Geometry: final body of the model. Coordinates: model frame, mm. Round coordinates to 2 decimals unless told otherwise and drop trailing zeros. Loops run counter-clockwise (first coordinate to the right, second up) from the corner with the lowest first, then second, coordinate; pieces in that order, holes last. Notation, with made-up numbers: M 69,-26 L 83,-26 A8 cw 83,-20 Z; hole C 15.25,-26.5 d6. An arc over 180 degrees is marked long. Return JSON: item names as keys, results as strings.
from build123d import *

# Parameters (mm, degrees)
F0_R        = 51.2
F1_DEPTH    = 1.5
F2_T1_DEPTH = 3
F3_R        = 5.08


# Not quite as in the source:
# - a fillet or chamfer that OpenCascade refuses, or shapes differently, is made with other operations: its cross-section is extruded or revolved along the edge and cut away or added


with BuildPart() as f1:
    # F0 (on Front) → F1 (new body, symmetric)
    with BuildSketch(Plane.XZ):
        Circle(F0_R)
        with BuildLine():
            ThreePointArc((1.5, 44.1745401787), (25.9801081513, 35.7585511514), (41.5489587997, 15.0772684084))
            ThreePointArc((41.5489587997, 15.0772684084), (42.0366980202, 13.6585511514), (42.4760097829, 12.2240988595))
            ThreePointArc((42.4760097829, 12.2240988595), (43.7668803572, 6.1725346333), (44.2, 0))
            ThreePointArc((44.2, 0), (39.7173586616, -19.3951391062), (27.1786687354, -34.8562758448))
            ThreePointArc((27.1786687354, -34.8562758448), (25.9801081513, -35.7585511514), (24.7516177523, -36.6196316017))
            ThreePointArc((24.7516177523, -36.6196316017), (0, -44.2), (-24.7516177523, -36.6196316017))
            ThreePointArc((-24.7516177523, -36.6196316017), (-25.9801081513, -35.7585511514), (-27.1786687354, -34.8562758448))
            ThreePointArc((-27.1786687354, -34.8562758448), (-42.0366980202, -13.6585511514), (-42.4760097829, 12.2240988595))
            ThreePointArc((-42.4760097829, 12.2240988595), (-42.0366980202, 13.6585511514), (-41.5489587997, 15.0772684084))
            ThreePointArc((-41.5489587997, 15.0772684084), (-25.9801081513, 35.7585511514), (-1.5, 44.1745401787))
            ThreePointArc((-1.5, 44.1745401787), (0, 44.2), (1.5, 44.1745401787))
        make_face(mode=Mode.SUBTRACT)
        with BuildLine():
            Line((-24.7516177523, -36.6196316017), (-1.118469097, -4.8732973313))
            ThreePointArc((-1.118469097, -4.8732973313), (-2.9389262615, -4.0450849719), (-4.2891552241, -2.569659017))
            Line((-4.2891552241, -2.569659017), (-27.1786687354, -34.8562758448))
            ThreePointArc((-27.1786687354, -34.8562758448), (-25.9801081513, -35.7585511514), (-24.7516177523, -36.6196316017))
        make_face()
        with BuildLine():
            ThreePointArc((-4.9804071414, -0.4422043711), (-4.7552825815, 1.5450849719), (-3.7693128085, 3.2851607193))
            Line((-3.7693128085, 3.2851607193), (-41.5489587997, 15.0772684084))
            ThreePointArc((-41.5489587997, 15.0772684084), (-42.0366980202, 13.6585511514), (-42.4760097829, 12.2240988595))
            Line((-42.4760097829, 12.2240988595), (-4.9804071414, -0.4422043711))
        make_face()
        with BuildLine():
            ThreePointArc((-1.9595917942, 4.6), (0, 5), (1.9595917942, 4.6))
            Line((1.9595917942, 4.6), (1.5, 44.1745401787))
            ThreePointArc((1.5, 44.1745401787), (0, 44.2), (-1.5, 44.1745401787))
            Line((-1.5, 44.1745401787), (-1.9595917942, 4.6))
        make_face()
        with BuildLine():
            ThreePointArc((3.7693128085, 3.2851607193), (4.6822304537, 1.7540575757), (5, 0))
            ThreePointArc((5, 0), (4.9950993837, -0.2213191055), (4.9804071414, -0.4422043711))
            Line((4.9804071414, -0.4422043711), (42.4760097829, 12.2240988595))
            ThreePointArc((42.4760097829, 12.2240988595), (42.0366980202, 13.6585511514), (41.5489587997, 15.0772684084))
            Line((41.5489587997, 15.0772684084), (3.7693128085, 3.2851607193))
        make_face()
        with BuildLine():
            Line((27.1786687354, -34.8562758448), (4.2891552241, -2.569659017))
            ThreePointArc((4.2891552241, -2.569659017), (2.9389262615, -4.0450849719), (1.118469097, -4.8732973313))
            Line((1.118469097, -4.8732973313), (24.7516177523, -36.6196316017))
            ThreePointArc((24.7516177523, -36.6196316017), (25.9801081513, -35.7585511514), (27.1786687354, -34.8562758448))
        make_face()
        with BuildLine():
            ThreePointArc((4.9804071414, -0.4422043711), (4.9950993837, -0.2213191055), (5, 0))
            ThreePointArc((5, 0), (4.6822304537, 1.7540575757), (3.7693128085, 3.2851607193))
            ThreePointArc((3.7693128085, 3.2851607193), (2.9389262615, 4.0450849719), (1.9595917942, 4.6))
            ThreePointArc((1.9595917942, 4.6), (0, 5), (-1.9595917942, 4.6))
            ThreePointArc((-1.9595917942, 4.6), (-2.9389262615, 4.0450849719), (-3.7693128085, 3.2851607193))
            ThreePointArc((-3.7693128085, 3.2851607193), (-4.7552825815, 1.5450849719), (-4.9804071414, -0.4422043711))
            ThreePointArc((-4.9804071414, -0.4422043711), (-4.7552825815, -1.5450849719), (-4.2891552241, -2.569659017))
            ThreePointArc((-4.2891552241, -2.569659017), (-2.9389262615, -4.0450849719), (-1.118469097, -4.8732973313))
            ThreePointArc((-1.118469097, -4.8732973313), (0, -5), (1.118469097, -4.8732973313))
            ThreePointArc((1.118469097, -4.8732973313), (2.9389262615, -4.0450849719), (4.2891552241, -2.569659017))
            ThreePointArc((4.2891552241, -2.569659017), (4.7552825815, -1.5450849719), (4.9804071414, -0.4422043711))
        make_face()
        with BuildLine():
            ThreePointArc((0, 1.5), (1.0606601718, 1.0606601718), (1.5, 0))
            ThreePointArc((1.5, 0), (-1.0606601718, -1.0606601718), (0, 1.5))
        make_face(mode=Mode.SUBTRACT)
    extrude(amount=F1_DEPTH, both=True)

    # F2: fillet of radius 3 on 10 edges, made by hand

    # F2_s2 → F2_t1 (join)
    with BuildSketch(Plane.XZ.offset(-1.5)):
        with BuildLine():
            ThreePointArc((3.0875868977, 3.9327861815), (2.2498717307, 4.9648804635), (1.9403413197, 6.2576202799))
            Line((1.9403413197, 6.2576202799), (1.9595917942, 4.6))
            ThreePointArc((1.9595917942, 4.6), (2.5455444913, 4.303510572), (3.0875868977, 3.9327861815))
        make_face()
        with BuildLine():
            ThreePointArc((2.7861851021, 4.151767404), (4.0266333175, 3.6739876086), (5.351752101, 3.7790852667))
            Line((5.351752101, 3.7790852667), (3.7693128085, 3.2851607193))
            ThreePointArc((3.7693128085, 3.2851607193), (3.3062652647, 3.7508145781), (2.7861851021, 4.151767404))
        make_face()
        with BuildLine():
            ThreePointArc((-2.7861851021, 4.151767404), (-4.0266333175, 3.6739876086), (-5.351752101, 3.7790852667))
            Line((-5.351752101, 3.7790852667), (-3.7693128085, 3.2851607193))
            ThreePointArc((-3.7693128085, 3.2851607193), (-3.3062652647, 3.7508145781), (-2.7861851021, 4.151767404))
        make_face()
        with BuildLine():
            ThreePointArc((-3.0875868977, 3.9327861815), (-2.2498717307, 4.9648804635), (-1.9403413197, 6.2576202799))
            Line((-1.9403413197, 6.2576202799), (-1.9595917942, 4.6))
            ThreePointArc((-1.9595917942, 4.6), (-2.5455444913, 4.303510572), (-3.0875868977, 3.9327861815))
        make_face()
        with BuildLine():
            ThreePointArc((-4.6944187481, -1.7211718734), (-5.4171305174, -0.605522732), (-6.5509489863, 0.0883367549))
            Line((-6.5509489863, 0.0883367549), (-4.9804071414, -0.4422043711))
            ThreePointArc((-4.9804071414, -0.4422043711), (-4.8794982801, -1.0910987737), (-4.6944187481, -1.7211718734))
        make_face()
        with BuildLine():
            ThreePointArc((-4.8095439897, -1.3668528124), (-4.7384679811, -2.6942312472), (-5.2479060175, -3.9220171386))
            Line((-5.2479060175, -3.9220171386), (-4.2891552241, -2.569659017))
            ThreePointArc((-4.2891552241, -2.569659017), (-4.5889288007, -1.9853796772), (-4.8095439897, -1.3668528124))
        make_face()
        with BuildLine():
            ThreePointArc((4.6944187481, -1.7211718734), (5.4171305174, -0.605522732), (6.5509489863, 0.0883367549))
            Line((6.5509489863, 0.0883367549), (4.9804071414, -0.4422043711))
            ThreePointArc((4.9804071414, -0.4422043711), (4.8794982801, -1.0910987737), (4.6944187481, -1.7211718734))
        make_face()
        with BuildLine():
            ThreePointArc((4.8095439897, -1.3668528124), (4.7384679811, -2.6942312472), (5.2479060175, -3.9220171386))
            Line((5.2479060175, -3.9220171386), (4.2891552241, -2.569659017))
            ThreePointArc((4.2891552241, -2.569659017), (4.5889288007, -1.9853796772), (4.8095439897, -1.3668528124))
        make_face()
        with BuildLine():
            ThreePointArc((0.186276554, -4.9965288997), (-1.0980990506, -5.3391140929), (-2.1083678125, -6.2030251629))
            Line((-2.1083678125, -6.2030251629), (-1.118469097, -4.8732973313))
            ThreePointArc((-1.118469097, -4.8732973313), (-0.4701512939, -4.9778466992), (0.186276554, -4.9965288997))
        make_face()
        with BuildLine():
            ThreePointArc((2.1083678125, -6.2030251629), (1.0980990506, -5.3391140929), (-0.186276554, -4.9965288997))
            ThreePointArc((-0.186276554, -4.9965288997), (0.4701512939, -4.9778466992), (1.118469097, -4.8732973313))
            Line((1.118469097, -4.8732973313), (2.1083678125, -6.2030251629))
        make_face()
    extrude(amount=F2_T1_DEPTH)

    # F3
    f3_edges = [f1.edges().sort_by_distance(p)[0] for p in [
        (-42.47601, 0, 12.224099),
        (42.47601, 0, 12.224099),
        (-1.5, 0, 44.17454),
        (24.751618, 0, -36.619632),
        (27.178669, 0, -34.856276),
        (41.548959, 0, 15.077268),
        (1.5, 0, 44.17454),
        (-41.548959, 0, 15.077268),
        (-27.178669, 0, -34.856276),
        (-24.751618, 0, -36.619632),
    ]]
    fillet(f3_edges, radius=F3_R)


solid = f1.part
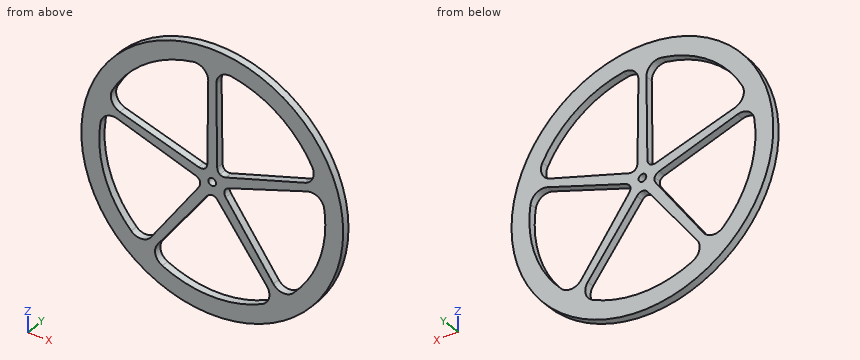
Q1. Section query B-B (x = -29). Output: boundary loops of the cut face in (y, z), plus the area to 3 significant figures.
Determined:
{"outline": "M -1.5,-42.2 L 1.5,-42.2 L 1.5,-32.27 L -1.5,-32.27 Z; M -1.5,7.67 L 1.5,7.67 L 1.5,11.16 L -1.5,11.16 Z; M -1.5,33.36 L 1.5,33.36 L 1.5,42.2 L -1.5,42.2 Z", "area": "66.8 mm^2"}
Q2. Pin query (flat end, axial travel): pin 1 (8 mm diameter, centred on x = -18.5, z = -33.5, fed in from -Y); pin 2 (1.5 mm diameter, centred on x = 30.5, y = -1, fed in from -Z). Return the tip coordinate at first contact, or that it passes through.
Determined:
{"pin 1": "stops at y = -1.5", "pin 2": "stops at z = -41.67"}
Q3. Section query A-A (z = -8.5). Output: boundary loops of the cut face in (x, y) (1 decimal), plus the area to 3 significant figures.
Determined:
{"outline": "M -50.5,-1.5 L -43.4,-1.5 L -43.4,1.5 L -50.5,1.5 Z; M -8.5,-1.5 L -3.8,-1.5 L -3.8,1.5 L -8.5,1.5 Z; M 3.8,-1.5 L 8.5,-1.5 L 8.5,1.5 L 3.8,1.5 Z; M 43.4,-1.5 L 50.5,-1.5 L 50.5,1.5 L 43.4,1.5 Z", "area": "70.7 mm^2"}
Q4. Section query D-D (y = -0.75). State how many separate pieces and enclosed holes the cut face has, plus the area to 3 significant figures.
Determined:
{"separate pieces": "1", "enclosed holes": "6", "area": "2,930 mm^2"}
Q5. Material intervals for L1, parallel to Z at x = -14, y = -1.35; L2, parallel to X at y = 1.35, z = -12; L3, parallel to Z at x = 30, y = -1.4, sorted ascending.
Determined:
{"L1": "z = -49.25 to -41.92, -22.18 to -16.27, 2.6 to 6.48, 41.92 to 49.25", "L2": "x = -49.77 to -42.54, -10.97 to -6.42, 6.42 to 10.97, 42.54 to 49.77", "L3": "z = -41.49 to -31.97, 8.01 to 11.47, 32.46 to 41.49"}
Q6. Section query C-C (z = 23). Output: boundary loops of the cut face in (x, y).
Determined:
{"outline": "M -45.74,-1.5 L -37.74,-1.5 L -37.74,1.5 L -45.74,1.5 Z; M -1.75,-1.5 L 1.75,-1.5 L 1.75,1.5 L -1.75,1.5 Z; M 37.74,-1.5 L 45.74,-1.5 L 45.74,1.5 L 37.74,1.5 Z"}
